Part model, mm, in its own coordinate system. A direction names the side the tool comes from. Give positions to 0.01 mm unless a question says otherwise; leave off trailing zeros. Order: outer loops, then holes, each group sorted by start corner. A loop starts at its lowest first (then second) coordinate and runs counter-clockwise, first axis right, second up.
1. Mould opens along X. For faces 4 (the flat face through (3.3, -54.5, 23)), 5 (the conical face through (-3.089, -65.155, 25.988)), 6 (the flat face through (-3.213, -61.553, 28.644)), 7 (the cylindrical face through (0.161, -47.549, 22.963)) say: +X half, -X half, draft (parallel to the pull), parting line (faces both ways), or undercut.
2. Which spindle directions (+Z, -Z, +X, -X, +Y, -Y) get a long thin tool onto all of the face, cutting with end or side? Do faces 1 (the flat face through (-3, -51, 25)), 2 (the flat face through (-2.7, -54.5, 28.9)), 3 (the flat face through (-2.56, -52.726, 23.154)). Say none if no direction does.
3. Slice it at A-A on y = -52.5. List the corners of the cut face in (x, z).
4. Probe line 1 (X direction, y = -59, z = 22.75); line 2 (X direction, y = -58.25, z = 26); line 3 (Y direction, x = 2.25, z = 25). List the from-to ranges inside material, lowest first.
5. Slice it at B-B on y = -50. List the corners of the cut face in (x, z), and give its area (3 significant figures).
6. Drop flat-ended pins along their axis: pin 1 Ø0.6 at (x, z) = (1, 25.5) entering from -Y; pin 2 Ø1.8 at (x, z) = (-3, 25) entering from -Y; pin 3 Ø0.8 at (x, z) = (0.5, 30) entering from -Y. Give the stop position or say it passes through.
from build123d import *

# Parameters (mm, degrees)
SKETCH005_R         = 3
PAD002_DEPTH        = 7
PAD003_DEPTH        = 3.5
SKETCH007_R         = 4
PAD004_DEPTH        = 8
FILLET_R            = 3
PAD005_DEPTH        = 2.5
BODY001_ROLL_ANGLE  = -180
BODY001_PITCH_ANGLE = 75


with BuildPart() as part:
    # Sketch005 → Pad002 (new body)
    with BuildSketch(Plane.XZ):
        Circle(SKETCH005_R)
    extrude(amount=PAD002_DEPTH)

    # Sketch006 (on Face2 of Pad002) → Pad003 (join)
    with BuildSketch(Plane(origin=(0, 0, 0), x_dir=(1, 0, 0), z_dir=(0, 1, 0))):
        Polygon((4, -2.3094010768), (4, 2.3094010768), (0, 4.6188021535), (-4, 2.3094010768), (-4, -2.3094010768), (0, -4.6188021535), align=None)
    extrude(amount=PAD003_DEPTH)

    # Sketch007 (on Face5 of Pad003) → Pad004 (join)
    with BuildSketch(Plane(origin=(0, 3.5, 0), x_dir=(1, 0, 0), z_dir=(0, 1, 0))):
        Circle(SKETCH007_R)
    extrude(amount=PAD004_DEPTH)

    # Fillet
    fillet_edges = [part.edges().sort_by_distance(p)[0] for p in [
        (-4, 11.5, 0),
    ]]
    fillet(fillet_edges, radius=FILLET_R)

    # Sketch008 (on Plane of DatumPlane) → Pad005 (join)
    with BuildSketch(Plane(origin=(0, 11.5, 0), x_dir=(1, 0, 0), z_dir=(0, 0.7071067812, 0.7071067812))):
        Polygon((3.5, -4.6207259421), (3.5, -0.5792740579), (0, 1.4414518843), (-3.5, -0.5792740579), (-3.5, -4.6207259421), (0, -6.6414518843), align=None)
    extrude(amount=PAD005_DEPTH)

    # Sketch009 (on Plane of DatumPlane001) → Revolution (revolve)
    with BuildSketch(Plane(origin=(0, 7.517766953, 7.517766953), x_dir=(0, -0.7071067812, -0.7071067812), z_dir=(1, 0, 0))):
        Polygon((0, 8.4317279836), (-2, 7.7817279836), (-3.5, 8.7817279836), (-4, 8.7817279836), (-5.5, 7.7817279836), (-5.5, 5.5317279836), (0, 5.5317279836), align=None)
    revolve(axis=Axis((0, 11.4292893219, 3.6062445841), (0, -0.7071067812, -0.7071067812)))


with BuildPart() as part_1:
    # Body001 roll: moved
    add(part.part.rotate(Axis((0, 0, 0), (1, 0, 0)), BODY001_ROLL_ANGLE))


with BuildPart() as part_2:
    # Body001 pitch: moved
    add(part_1.part.rotate(Axis((0, 0, 0), (0, 1, 0)), BODY001_PITCH_ANGLE))


with BuildPart() as part_3:
    # Body001 placement: moved
    add(part_2.part.moved(Location((0.2910046565, -51, 25.9598789729))))


solid = part_3.part
Data:
1. face 4: draft
1. face 5: undercut
1. face 6: -X half
1. face 7: parting line
2. face 1: +Y
2. face 2: +Z, -X
2. face 3: -Z, -X, +Y
3. outline: (-4.17, 24.76) - (-0.9, 21.5) - (3.56, 22.69) - (4.75, 27.16) - (1.49, 30.42) - (-2.97, 29.23) - close
4. line 1: x = -3.06 to -2.47, -2.1 to 2.68
4. line 2: x = -3.71 to 4.29
4. line 3: y = -62.26 to -44
5. outline: circle Ø6 at (0.29, 25.96)
5. area: 28.3 mm2
6. pin 1: stops at y = -63.85
6. pin 2: stops at y = -67.59
6. pin 3: stops at y = -60.91
